Geometry check sheet. Reference: the model listing, model coordinates, mm. Round coordinates to 2 decimals unless told otherwise and drop trailing zeros. Order: outer loops, then holes, each group sorted by start corner. A loop starts at its lowest first (then second) coordinate and runs counter-clockwise, first axis right, second up. Notation, with made-up numbers: M 69,-3 L 106,-3 A22 ccw 106,19 Z; hole C 47.5,-19 d6. An arc over 180 degrees is marked long. Answer as a JSON object with one key per item and string values. Group by question number.
```python
from build123d import *

# Parameters (mm, degrees)
BOSS_EXTRUDE1_DEPTH = 60
SKETCH3_W           = 31.691445316
SKETCH3_H           = 5
CUT_EXTRUDE1_DEPTH  = 63.561969278


with BuildPart() as part:
    # Sketch1 → Boss-Extrude1 (new body)
    with BuildSketch(Plane(origin=(0, 0, 0), x_dir=(0, 0, -1), z_dir=(1, 0, 0))):
        with BuildLine():
            Line((0, -2.5), (17, -2.5))
            Line((17, -2.5), (17, -0.5))
            Line((17, -0.5), (2.449489743, -0.5))
            ThreePointArc((2.449489743, -0.5), (-1.58113883, 1.936491673), (0, -2.5))
        make_face()
    extrude(amount=BOSS_EXTRUDE1_DEPTH)

    # Sketch3 → Cut-Extrude1 (cut, through all)
    with BuildSketch(Plane.XZ.offset(2.5)):
        with Locations((45.845722658, 0)):
            Rectangle(SKETCH3_W, SKETCH3_H)
    extrude(amount=-CUT_EXTRUDE1_DEPTH, mode=Mode.SUBTRACT)


solid = part.part
```
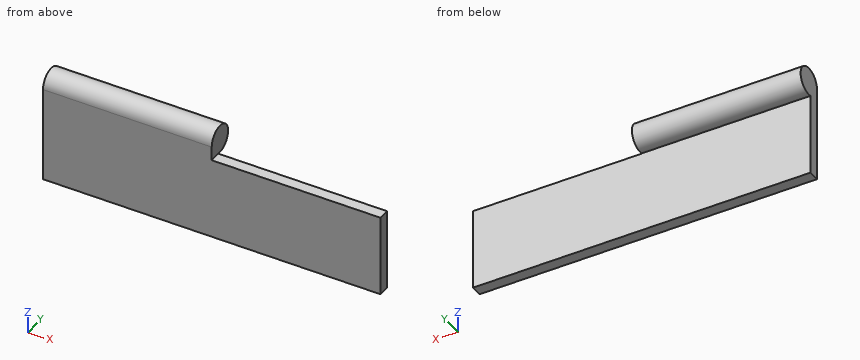
1) Sectioned sample at B-B (z = -10.5). Record the boundary of the cut face in (x, y).
2) Sectioned sample at A-A (x = 55). Record the boundary of the cut face in (y, z).
3) Go/stop test with flat-tipped pins: P1, Ø1.5, axis at x = 7, z = -12, coming from the +Y side; P2, Ø2, axis at x = 49.5, y = -1.5, coming from the +Z side; P3, Ø11.5, axis at x = 22.5, z = -8, coming from the +Y side. Record where each tip stops, or that it passes through.
4) Sectioned sample at C-C (y = -1.9). Record the boundary of the cut face in (x, z).
5) Thickness scan on line 1 along Y through (x, z) = (12, -11.75); line 2 along Z through (x, y) = (6.5, -0.05); line 3 along X through (y, z) = (-0.8, -0.75). Record the ranges inside material, lowest first. Write a range as [from, to].
Final values:
{
 "1": {"outline": "M 0,-2.5 L 60,-2.5 L 60,-0.5 L 0,-0.5 Z"},
 "2": {"outline": "M -2.5,-17 L -0.5,-17 L -0.5,-2.5 L -2.5,-2.5 Z"},
 "3": {"P1": "stops at y = -0.5", "P2": "stops at z = -2.5", "P3": "stops at y = 1.09"},
 "4": {"outline": "M 0,-17 L 60,-17 L 60,-2.5 L 30,-2.5 L 30,1.62 L 0,1.62 Z"},
 "5": {"line 1": "y = [-2.5, -0.5]", "line 2": "z = [-2.5, 2.5]", "line 3": "x = [0, 30]"}
}
